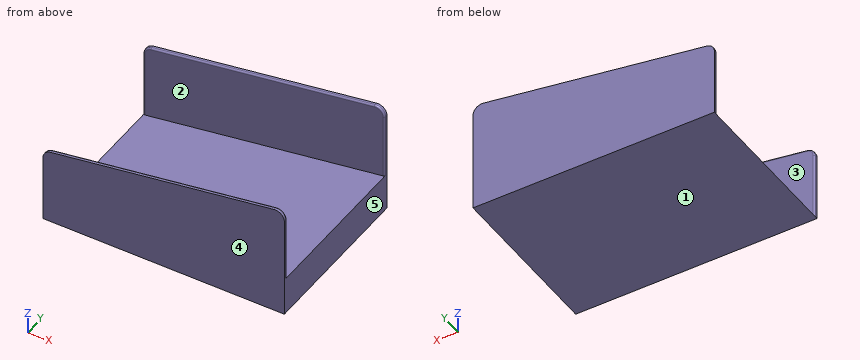
```python
from build123d import *

# Parameters (mm, degrees)
F0_W     = 203.2
F0_H     = 133.35
F1_DEPTH = 31.75
F3_DEPTH = 133.35
F4_W     = 203.2
F4_H     = 3.175
F5_DEPTH = 95.25
F7_DEPTH = 139.7
F8_R     = 7.62
F9_R     = 1.27


with BuildPart() as f1:
    # F0 (on Top) → F1 (new body)
    with BuildSketch(Plane.XY):
        Rectangle(F0_W, F0_H)
    extrude(amount=F1_DEPTH)

    # F2 (on face) → F3 (cut, through all)
    with BuildSketch(Plane.XZ.offset(66.675)):
        Polygon((-101.6, 31.75), (-101.6, 0), (101.6, 31.75), align=None)
    extrude(amount=-F3_DEPTH, mode=Mode.SUBTRACT)

    # F4 (on Top) → F5 (join)
    with BuildSketch(Plane.XY):
        with Locations((0, 68.2625)):
            Rectangle(F4_W, F4_H)
        with Locations((0, -68.2625)):
            Rectangle(F4_W, F4_H)
    extrude(amount=F5_DEPTH)

    # F6 (on face) → F7 (cut, through all)
    with BuildSketch(Plane.XZ.offset(69.85)):
        Polygon((-101.6, 63.5), (101.6, 95.25), (-101.6, 95.25), align=None)
    extrude(amount=-F7_DEPTH, mode=Mode.SUBTRACT)

    # F8
    f8_edges = [f1.edges().sort_by_distance(p)[0] for p in [
        (101.6, -68.2625, 95.25),
        (101.6, 68.2625, 95.25),
        (-101.6, -68.2625, 63.5),
        (-101.6, 68.2625, 63.5),
    ]]
    fillet(f8_edges, radius=F8_R)

    # F9
    f9_edges = [f1.edges().sort_by_distance(p)[0] for p in [
        (101.6, -66.675, 59.048459),
        (101.6, 66.675, 59.048459),
    ]]
    fillet(f9_edges, radius=F9_R)


solid = f1.part
```
Design review of the part built by this model. Coordinates are the model's own, in mm. Face numbers are marked on the shaded views. A direction names the side the tool comes from. Give positions to 0.01 mm unless a question says otherwise; leave off trailing zeros. Write each loop counter-clockwise with the first axis right and the second up, starting at its lowest first coordinate (ties: lowest second). Pieces come first, ordered by that corner, then holes. Notation, with made-up numbers: (20, -30) -> (28, -30) arc R15 cw to (28, -14) -> close; hole circle Ø3 at (-27, 38.5). An arc over 180 degrees is marked (long way). Answer in a Markdown table with one row per item.
(1) Consider section A-A (z = 45). State the section outline as (x, y) points (3 decimals), then the cut area to 3 significant figures.
Results:
| item | result |
|---|---|
| outline | (-101.6, -69.85) -> (101.6, -69.85) -> (101.6, -67.945) arc R1.27 ccw to (100.33, -66.675) -> (-100.33, -66.675) arc R1.27 ccw to (-101.6, -67.945) -> close; (-101.6, 67.945) arc R1.27 ccw to (-100.33, 66.675) -> (100.33, 66.675) arc R1.27 ccw to (101.6, 67.945) -> (101.6, 69.85) -> (-101.6, 69.85) -> close |
| area | 1,290 mm2 |
(2) Consider section B-B (z = 20.5). State the section outline as (x, y) points (3 decimals), then the cut area to 3 significant figures.
Results:
| item | result |
|---|---|
| outline | (-101.6, -69.85) -> (101.6, -69.85) -> (101.6, 69.85) -> (-101.6, 69.85) -> (-101.6, 67.945) arc R1.27 ccw to (-100.33, 66.675) -> (29.6, 66.675) -> (29.6, -66.675) -> (-100.33, -66.675) arc R1.27 ccw to (-101.6, -67.945) -> close |
| area | 10,900 mm2 |
(3) Clearance check with a flat-ended pin moving along its axis: pin 1 (12 mm diameter, centred on x = 49, y = 55, fed in from +Z). State where the tip first meets the part, or that it passes through.
Results:
| item | result |
|---|---|
| pin 1 | z = 24.47 |
(4) Mouldability with a two-part tool opening along Y and no side actions: class the marked faces 3, 4 and 5 as +Y half, -Y half, draft (parallel to the pull), parting line (faces both ways), or undercut.
Results:
| item | result |
|---|---|
| face 3 | undercut |
| face 4 | -Y half |
| face 5 | draft |
(5) Consider section C-C (y = 36.5). State the section outline as (x, z) points.
Results:
| item | result |
|---|---|
| outline | (-101.6, 0) -> (101.6, 0) -> (101.6, 31.75) -> close |
(6) For the marked faces 1 and 2, list the 3-axis set-ups (+Z, -Z, +X, -X, +Y, -Y) from which the entire face can be reached by the end or side of a thin tool; tool diameter is ignored.
Results:
| item | result |
|---|---|
| face 1 | -Z, +X, -X, +Y, -Y |
| face 2 | +Z, -X |
(7) To check wall thickness, follow probe 1 along Y at (x, z) = (-21.5, 19) (3 decimals); probe 2 along Z at (x, y) = (-38.5, 63.5). State the ranges of each line that lie inside material, in increasing order.
Results:
| item | result |
|---|---|
| probe 1 | -69.85 to -66.675, 66.675 to 69.85 |
| probe 2 | 0 to 9.86 |
